CAD build for the part. Positions are in the model's coordinates, mm. A direction names the side the tool comes from. Round coordinates to 2 decimals unless told otherwise and drop trailing zeros. Order: outer loops, then holes, each group sorted by start corner. A loop starts at its lowest first (then second) coordinate and runs counter-clockwise, first axis right, second up. Notation, with made-up numbers: (33.5, 66.25) - (49.5, 66.25) arc R28 cw to (49.5, 98.25) - close; hole circle Ø9 at (88, 65). An arc over 180 degrees is marked (long way). Write item = value, one per line.
from build123d import *

# Parameters (mm, degrees)
SKETCH_1_W          = 10
SKETCH_1_H          = 10
SKETCH_1_W_2        = 8
SKETCH_1_H_2        = 8
EXTRUDE_1_DEPTH     = 85
SKETCH_2_R          = 1.5
CUT_EXTRUDE_1_DEPTH = 11
SKETCH_3_R          = 1.5
CUT_EXTRUDE_2_DEPTH = 10
SKETCH_4_R          = 3.5
CUT_EXTRUDE_3_DEPTH = 5
FILLET_1_R          = 0.5


with BuildPart() as part:
    # 草图1 → 拉伸-薄壁1 (new body)
    with BuildSketch(Plane.XY):
        Rectangle(SKETCH_1_W, SKETCH_1_H)
        Rectangle(SKETCH_1_W_2, SKETCH_1_H_2, mode=Mode.SUBTRACT)
    extrude(amount=EXTRUDE_1_DEPTH)

    # 草图2 → 切除-拉伸1 (cut, through all)
    with BuildSketch(Plane(origin=(0, 5, 0), x_dir=(1, 0, 0), z_dir=(0, 1, 0))):
        with Locations((0, -70)):
            Circle(SKETCH_2_R)
        with Locations((0, -5)):
            Circle(SKETCH_2_R)
        with Locations((0, -30)):
            Circle(SKETCH_2_R)
    extrude(amount=-CUT_EXTRUDE_1_DEPTH, mode=Mode.SUBTRACT)

    # 草图3 → 切除-拉伸2 (cut)
    with BuildSketch(Plane.ZY.offset(5)):
        with Locations((25, 0)):
            Circle(SKETCH_3_R)
        with Locations((60, 0)):
            Circle(SKETCH_3_R)
        with Locations((80, 0)):
            Circle(SKETCH_3_R)
    extrude(amount=-CUT_EXTRUDE_2_DEPTH, mode=Mode.SUBTRACT)

    # 草图4 → 切除-拉伸3 (cut)
    with BuildSketch(Plane(origin=(0, 5, 0), x_dir=(1, 0, 0), z_dir=(0, 1, 0))):
        with Locations((0, -5)):
            Circle(SKETCH_4_R)
        with Locations((0, -30)):
            Circle(SKETCH_4_R)
        with Locations((0, -70)):
            Circle(SKETCH_4_R)
    extrude(amount=-CUT_EXTRUDE_3_DEPTH, mode=Mode.SUBTRACT)

    # 圆角1
    fillet_1_edges = [part.edges().sort_by_distance(p)[0] for p in [
        (5, 0, 0),
        (-5, 0, 0),
    ]]
    fillet(fillet_1_edges, radius=FILLET_1_R)


solid = part.part
(1) Tool access for faces 1 (the cylindrical face through (-0.46, 4.51, 26.53)), 2 (the flat face through (4, 0, 42)), 3 (the cylindrical face through (4.49, 0.45, 81.43)): list every direction of +Z, -Z, +X, -X, +Y, -Y with a clear straight run to the whole face (end or side of a thin tool).
Solved:
face_1 = +Y
face_2 = +Z, -Z
face_3 = +X, -X
(2) Band-saw the part on A-A on x = 0. Count the separate pieces of the cut face and the enclosed holes in it, plus the area to 3 significant figures.
Solved:
separate_pieces = 8
enclosed_holes = 0
area = 140 mm²
(3) Band-saw the part on B-B on z = 25. List the corners of the cut face in (x, y).
Solved:
outline = (-5, -5) - (5, -5) - (5, -1.5) - (4, -1.5) - (4, -4) - (-4, -4) - (-4, -1.5) - (-5, -1.5) - close; (-5, 1.5) - (-4, 1.5) - (-4, 4) - (4, 4) - (4, 1.5) - (5, 1.5) - (5, 5) - (-5, 5) - close
(4) Probe line 1 along Z through (x, y) = (0, 4.55); line 2 along Y through (x, z) = (4.7, 25); line 3 along Y through (x, z) = (2.5, 51). List the from-to ranges inside material, lowest first.
Solved:
line_1 = 0 to 1.5, 8.5 to 26.5, 33.5 to 66.5, 73.5 to 85
line_2 = -5 to -1.5, 1.5 to 5
line_3 = -5 to -4, 4 to 5
(5) Pull direction Y, two halves, no side cores. Call faces 4 (the flat face through (0, -5, 42)), 5 (the cylindrical face through (0.806, -4.493, 68.735)), 6 (the flat face through (-4, 0, 42)): released by +Y, released by -Y, zero draft, split by the parting line, or undercut.
Solved:
face_4 = released by -Y
face_5 = zero draft
face_6 = undercut
(6) Drop flat-ended pins along their axis: pin 1 (2.5 mm diameter, centred on y = 0, z = 25, fed in from +X); pin 2 (4 mm diameter, centred on x = 0, z = 5, fed in from +Y). Give the stop position or say it passes through.
Solved:
pin_1 = through
pin_2 = -4
(7) Band-saw the part on C-C on y = 3.25. List the corners of the cut face in (x, z), plus the area to 3 significant figures.
Solved:
outline = (-5, 0.5) arc R0.5 ccw to (-4.5, 0) - (-4, 0) - (-4, 85) - (-5, 85) - close; (4, 0) - (4.5, 0) arc R0.5 ccw to (5, 0.5) - (5, 85) - (4, 85) - close
area = 170 mm²
